Here's how the part is built. I have some questions about the finished solid (model axes, mm). Face numbers are marked on the shaded views. A direction names the side the tool comes from. Give positions to 0.01 mm unless a question says otherwise; leave off trailing zeros. Loops run counter-clockwise (first coordinate to the right, second up) from the corner with the lowest first, then second, coordinate; pieces in that order, holes last.
Q1. If we section it at C-C (y = 6.25): Please give me the cut outline in (x, z), plus the area to 3 significant figures.
Q2. I need wall thicknesses on line 1 (Z direction, x = -12.25, y = 2.75); line 2 (Y direction, x = -10, z = 5.5); line 3 (X direction, y = 6.5, z = 3). Which ranges of each line are inside material? Lowest first, please.
Q3. If we section it at B-B (x = -10.58): Please give me the cut outline in (y, z).
Q4. If we section it at D-D (z = 5.5): Please give me the cut outline in (x, y), plus the area to 3 significant figures.
Q5. Will this pin go through, and if not, where does the flat tip stop? P1, Ø1.6, axis at x = -6, y = 3.5, coming from the -Z side.
Q6. For the marked faces 1 and 2, which set-ups out of +Z, -Z, +X, -X, +Y, -Y let a thin tool reach every point of the face, with its end or its side?
Q7. If we section it at A-A (z = 3.44): Please give me the cut outline in (x, y).
Q8. We'd pull the mould along X, two halves only. Please class the marked faces 3, 4 and 5: +X half, -X half, draft (parallel to the pull), parting line (faces both ways), or undercut.
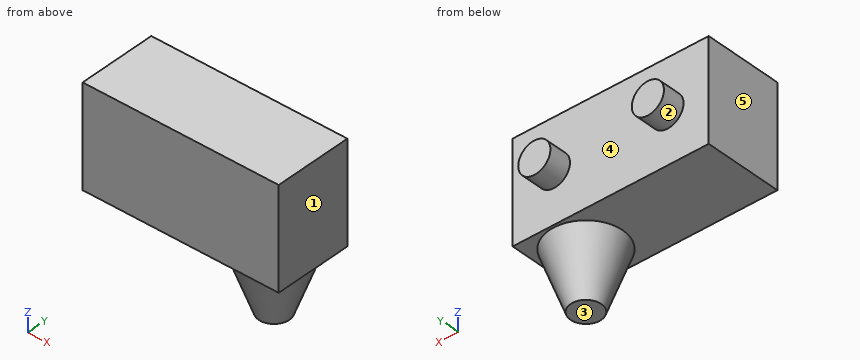
from build123d import *

# Parameters (mm, degrees)
SKETCH1_W           = 13.4
SKETCH1_H           = 5.33
BOSS_EXTRUDE1_DEPTH = 6.88
SKETCH2_R           = 1.1
BOSS_EXTRUDE2_DEPTH = 1.52
SKETCH3_R           = 2.5
BOSS_EXTRUDE3_DEPTH = 4
BOSS_EXTRUDE3_TAPER = 20


with BuildPart() as part:
    # Sketch1 → Boss-Extrude1 (new body)
    with BuildSketch(Plane.XY):
        with Locations((-6.7, 2.665)):
            Rectangle(SKETCH1_W, SKETCH1_H)
    extrude(amount=BOSS_EXTRUDE1_DEPTH)

    # Sketch2 → Boss-Extrude2 (add)
    with BuildSketch(Plane(origin=(0, 5.33, 0), x_dir=(1, 0, 0), z_dir=(0, 1, 0))):
        with Locations((-10.58, -3.44)):
            Circle(SKETCH2_R)
        with Locations((-2.82, -3.44)):
            Circle(SKETCH2_R)
    extrude(amount=BOSS_EXTRUDE2_DEPTH)

    # Sketch3 → Boss-Extrude3 (add)
    with BuildSketch(Plane(origin=(0, 0, 0), x_dir=(-1, 0, 0), z_dir=(0, 0, -1))):
        with Locations((2.665, 2.665)):
            Circle(SKETCH3_R)
    extrude(amount=BOSS_EXTRUDE3_DEPTH, taper=BOSS_EXTRUDE3_TAPER)


solid = part.part
Check sheet entries:
1. outline: circle Ø2.2 at (-10.58, 3.44); circle Ø2.2 at (-2.82, 3.44)
1. area: 7.60 mm2
2. line 1: z = 0 to 6.88
2. line 2: y = 0 to 5.33
2. line 3: x = -11.59 to -9.57, -3.83 to -1.81
3. outline: (0, 0) - (5.33, 0) - (5.33, 2.34) - (6.85, 2.34) - (6.85, 4.54) - (5.33, 4.54) - (5.33, 6.88) - (0, 6.88) - close
4. outline: (-13.4, 0) - (0, 0) - (0, 5.33) - (-13.4, 5.33) - close
4. area: 71.4 mm2
5. P1: stops at z = 0
6. face 1: +Z, -Z, +X, +Y, -Y
6. face 2: +Y
7. outline: (-13.4, 0) - (0, 0) - (0, 5.33) - (-1.72, 5.33) - (-1.72, 6.85) - (-3.92, 6.85) - (-3.92, 5.33) - (-9.48, 5.33) - (-9.48, 6.85) - (-11.68, 6.85) - (-11.68, 5.33) - (-13.4, 5.33) - close
8. face 3: draft
8. face 4: undercut
8. face 5: -X half
